CAD build for the part. Positions are in the model's coordinates, mm. A direction names the side the tool comes from. Give positions to 0.01 mm unless a question says otherwise; leave off trailing zeros. Order: outer loops, then holes, each group sorted by start corner. A loop starts at its lowest first (then second) coordinate and runs counter-clockwise, first axis right, second up.
Autodesk Fusion 360 part; units mm, degrees
sketch "Sketch1" plane through (0, 0, 0) normal (0, 1, 0) x (1, 0, 0)
  line L0 (0, 0) -> (103, 0)
  line L1 (103, 0) -> (103, 78.5)
  line L2 (103, 78.5) -> (0, 78.5)
  line L3 (0, 78.5) -> (0, 0)
  dimension "d1" = 103
  dimension "d2" = 78.5
extrude "Extrude1" add sketch "Sketch1" along normal blind 3
fillet "Fillet1" radius 3 4 edges at (0, 1.5, 0) (103, 1.5, 0) (103, 1.5, -78.5) (0, 1.5, -78.5)
sketch "Sketch6" plane through (0, 3, 0) normal (0, 1, 0) x (-1, 0, 0)
  arc A0 (-3, -78.5) -> (0, -75.5) centre (-3, -75.5) ccw
  line L0 (0, -75.5) -> (0, -3)
  arc A1 (0, -3) -> (-3, 0) centre (-3, -3) ccw
  line L1 (-3, 0) -> (-100, 0)
  arc A2 (-100, 0) -> (-103, -3) centre (-100, -3) ccw
  line L2 (-103, -3) -> (-103, -75.5)
  arc A3 (-103, -75.5) -> (-100, -78.5) centre (-100, -75.5) ccw
  line L3 (-100, -78.5) -> (-3, -78.5)
  line L4 (-1.5, -72.5) -> (-1.5, -6)
  line L5 (-1.5, -6) -> (-2.5, -6)
  line L6 (-2.5, -6) -> (-6, -3)
  line L7 (-6, -3) -> (-6, -2)
  line L8 (-6, -2) -> (-97, -2)
  line L9 (-97, -2) -> (-97, -3)
  line L10 (-97, -3) -> (-100, -6)
  line L11 (-100, -6) -> (-101, -6)
  line L12 (-101, -6) -> (-101, -72.5)
  line L13 (-101, -72.5) -> (-100, -72.5)
  line L14 (-100, -72.5) -> (-97, -75.5)
  line L15 (-97, -75.5) -> (-97, -76.5)
  line L16 (-97, -76.5) -> (-6, -76.5)
  line L17 (-6, -76.5) -> (-6.0056, -75.5)
  line L18 (-6.0056, -75.5) -> (-2.5, -72.4923)
  line L19 (-2.5, -72.4923) -> (-1.5, -72.5)
  dimension "d181" = 6
  dimension "d182" = 6
  dimension "d184" = 1
  dimension "d185" = 6
  dimension "d186" = 66.5
  dimension "d187" = 1
  dimension "d188" = 1
  dimension "d189" = 1
  dimension "d191" = 6
  dimension "d192" = 6
  dimension "d193" = 1
  dimension "d194" = 1
  dimension "d195" = 6
  dimension "d196" = 1
  dimension "d197" = 6
  dimension "d198" = 1
  dimension "d199" = 6
  dimension "d200" = 2
  dimension "d201" = 2
  dimension "d202" = 2
  dimension "d203" = 2
  dimension "d204" = 2
  dimension "d205" = 2
  dimension "d206" = 1.5
  dimension "d207" = 2
extrude "Extrude6" cut sketch "Sketch6" against normal blind 2 contours L4 L5 L6 L7 L8 L9 L10 L11 L12 L13 L14 L15 L16 L17 L18 L19
sketch "Sketch7" plane through (0, 3, 0) normal (0, 1, 0) x (-1, 0, 0)
  line L0 (-1.5, -6) -> (-1.5, -72.5)
  line L1 (-1.5, -72.5) -> (-2.5, -72.4923)
  line L2 (-2.5, -72.4923) -> (-6.0056, -75.5)
  line L3 (-6.0056, -75.5) -> (-6, -76.5)
  line L4 (-6, -76.5) -> (-97, -76.5)
  line L5 (-97, -76.5) -> (-97, -75.5)
  line L6 (-97, -75.5) -> (-100, -72.5)
  line L7 (-100, -72.5) -> (-101, -72.5)
  line L8 (-101, -72.5) -> (-101, -6)
  line L9 (-101, -6) -> (-100, -6)
  line L10 (-100, -6) -> (-97, -3)
  line L11 (-97, -3) -> (-97, -2)
  line L12 (-97, -2) -> (-6, -2)
  line L13 (-6, -2) -> (-6, -3)
  line L14 (-6, -3) -> (-2.5, -6)
  line L15 (-2.5, -6) -> (-1.5, -6)
  arc A0 (-3, -78.5) -> (0, -75.5) centre (-3, -75.5) ccw
  line L16 (0, -75.5) -> (0, -3)
  arc A1 (0, -3) -> (-3, 0) centre (-3, -3) ccw
  line L17 (-3, 0) -> (-100, 0)
  arc A2 (-100, 0) -> (-103, -3) centre (-100, -3) ccw
  line L18 (-103, -3) -> (-103, -75.5)
  arc A3 (-103, -75.5) -> (-100, -78.5) centre (-100, -75.5) ccw
  line L19 (-100, -78.5) -> (-3, -78.5)
  point P0 (-3, -75.5)
  point P1 (-100, -75.5)
  point P2 (-3, -3)
  point P3 (-100, -3)
hole "Hole1" at (3, 3, -75.5) at (100, 3, -75.5) at (3, 3, -3) at (100, 3, -3) direction (0, -1, 0) diameter 2.529 depth 2 tip angle 180
Item 1: Tool access for faces 5 (the face through (100, 1, -76)), 6 (the face through (0.86, 1.52, -0.9)): list every direction of +Z, -Z, +X, -X, +Y, -Y with a clear straight run to the whole face (end or side of a thin tool).
Item 2: Wall check: L1, parallel to X at y = 1.95, z = -3; L2, parallel to Z at x = 100, y = 1.45; L3, parallel to X at y = 1.1, z = -56. Give the ranges that are in metal, low to high.
Item 3: Slice it at B-B (z = -55.5). Give the cut face in (x, y), and give its area (3 significant figures).
Item 4: Slice it at C-C (x = 37). Give the cut face in (y, z), and give its area (3 significant figures).
Item 5: Two-plate mould, pull along X, no slides. Class faces 1 (the face through (102.14, 1.52, -77.6)), 2 (the face through (52, 1, -78.5)), 3 (the face through (52, 1, -39)), 4 (the face through (99.944, 1.986, -76.763)): released by +X, released by -X, zero draft, split by the parting line, or undercut.
Item 6: Drop flat-ended pins along their axis: pin 1 Ø1 at (x, z) = (51.5, -33) entering from +Y; pin 2 Ø0.5 at (x, y) = (2, 1.5) entering from -Z. Give the stop position or say it passes through.
Item 7: Slice it at A-A (y = 2.2). Give the cut face in (x, z).
A:
1. face 5: +Y
1. face 6: +Z, -X, +Y, -Y
2. L1: x = 0 to 1.74, 4.26 to 6, 97 to 98.74, 101.26 to 103
2. L2: z = -78.5 to -76.76, -74.24 to -72.5, -6 to -4.26, -1.74 to 0
2. L3: x = 0 to 1.5, 101 to 103
3. outline: (0, 0) - (103, 0) - (103, 3) - (101, 3) - (101, 1) - (1.5, 1) - (1.5, 3) - (0, 3) - close
3. area: 110 mm2
4. outline: (0, -78.5) - (3, -78.5) - (3, -76.5) - (1, -76.5) - (1, -2) - (3, -2) - (3, 0) - (0, 0) - close
4. area: 86.5 mm2
5. face 1: released by +X
5. face 2: zero draft
5. face 3: undercut
5. face 4: undercut
6. pin 1: stops at y = 1
6. pin 2: stops at z = -78.4
7. outline: (0, -75.5) arc R3 ccw to (3, -78.5) - (100, -78.5) arc R3 ccw to (103, -75.5) - (103, -3) arc R3 ccw to (100, 0) - (3, 0) arc R3 ccw to (0, -3) - close; hole (1.5, -72.5) - (2.5, -72.49) - (6.01, -75.5) - (6, -76.5) - (97, -76.5) - (97, -75.5) - (100, -72.5) - (101, -72.5) - (101, -6) - (100, -6) - (97, -3) - (97, -2) - (6, -2) - (6, -3) - (2.5, -6) - (1.5, -6) - close; hole circle Ø2.53 at (3, -75.5); hole circle Ø2.53 at (3, -3); hole circle Ø2.53 at (100, -75.5); hole circle Ø2.53 at (100, -3)
